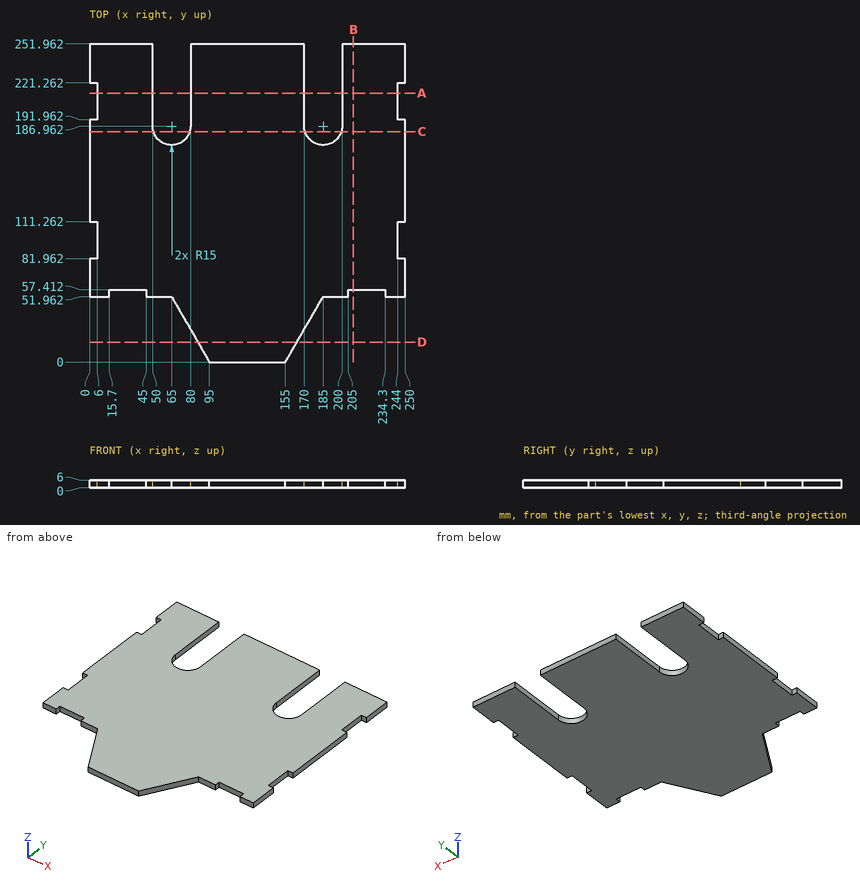
Here's the drawing with two shaded views (mm, measured from the low corner). I have some questions. Round coordinates to 2 decimals unless told otherwise and drop trailing zeros. Write each loop counter-clockwise with the first axis right and the second up, starting at its lowest first coordinate (ties: lowest second). Pieces come first, ordered by that corner, then holes. Notation, with made-up numbers: M 32,16 L 66,16 A15 cw 66,21 Z; hole C -5.5,17.25 d7. An arc over 180 degrees is marked long. Answer in a Markdown table with one row per item. Add a question column.
Q1. Imagine slicing it at A-A (y = 213). Please give me the cut outline in (x, z).
Q2. Imagine slicing it at D-D (y = 16). Please give me the cut outline in (x, z), then the cut area to 3 significant figures.
Q3. If I drill on line 1 (X direction, y = 239, z = 4.2); line 2 (X direction, y = 203.5, z = 3.95); line 3 (Y direction, x = 16.5, z = 2.2), over which ranges is the centre line in solid material (lowest first)? Write a range as from..to.
Q4. Imagine slicing it at C-C (y = 182.5). Please give me the cut outline in (x, z).
Q5. Imagine slicing it at B-B (x = 209). Please give me the cut outline in (y, z).
Q6. Will these pins go through, and if not, where does the flat tip stop? pin 1 Ø1.8 at (y, z) = (103, 3) entering from -X; pin 2 Ø1.8 at (y, z) = (219.5, 2) entering from +X; pin 3 Ø1.8 at (x, z) = (26, 4) entering from -Y.
Values:
| question | item | result |
|---|---|---|
| 1 | outline | M 6,0 L 50,0 L 50,6 L 6,6 Z; M 80,0 L 170,0 L 170,6 L 80,6 Z; M 200,0 L 244,0 L 244,6 L 200,6 Z |
| 2 | outline | M 85.76,0 L 164.24,0 L 164.24,6 L 85.76,6 Z |
| 2 | area | 471 mm^2 |
| 3 | line 1 | 0..50, 80..170, 200..250 |
| 3 | line 2 | 6..50, 80..170, 200..244 |
| 3 | line 3 | 57.41..251.96 |
| 4 | outline | M 0,0 L 50.68,0 L 50.68,6 L 0,6 Z; M 79.32,0 L 170.68,0 L 170.68,6 L 79.32,6 Z; M 199.32,0 L 250,0 L 250,6 L 199.32,6 Z |
| 5 | outline | M 57.41,0 L 251.96,0 L 251.96,6 L 57.41,6 Z |
| 6 | pin 1 | x = 6 |
| 6 | pin 2 | x = 244 |
| 6 | pin 3 | y = 57.41 |
